Autodesk Inventor part; units mm, degrees
ref_plane "YZ Plane" through (0, 0, 0) normal (1, 0, 0) x (0, 1, 0)
ref_plane "XZ Plane" through (0, 0, 0) normal (0, 1, 0) x (-1, 0, 0)
ref_plane "XY Plane" through (0, 0, 0) normal (0, 0, 1) x (1, 0, 0)
sketch "スケッチ1" plane through (0, 0, 0) normal (0, 1, 0) x (-1, 0, 0)
  line L0 (5.0263, 6.4044) -> (-44.9737, 6.4044)
  line L1 (-44.9737, 6.4044) -> (-44.9737, -43.5956)
  line L2 (-44.9737, -43.5956) -> (5.0263, -43.5956)
  line L3 (5.0263, -43.5956) -> (5.0263, 6.4044)
  point P0 (0, 0)
  dimension "d0" = 50
  dimension "d1" = 50
extrude "押し出し1" add sketch "スケッチ1" along normal blind 2
sketch "スケッチ2" plane through (0, 2, 0) normal (0, 1, 0) x (1, 0, 0)
  circle A0 centre (19.9737, 1.0956) radius 1.5
  line L0 (-5.0263, -6.4044) -> (44.9737, -6.4044)
  line L1 (-5.0263, 43.5956) -> (-5.0263, -6.4044)
  circle A1 centre (9.9737, 1.0956) radius 1.5
  circle A2 centre (29.9737, 1.0956) radius 1.5
  circle A3 centre (9.9737, 18.5956) radius 1.5
  circle A4 centre (19.9737, 18.5956) radius 1.5
  circle A5 centre (29.9737, 18.5956) radius 1.5
  point P0 (0, 0)
  dimension "d4" = 3
  dimension "d5" = 7.5
  dimension "d6" = 25
  dimension "d7" = 3
  dimension "d8" = 3
  dimension "d9" = 10
  dimension "d10" = 10
  dimension "d11" = 3
  dimension "d12" = 17.5
  dimension "d13" = 3
  dimension "d14" = 3
  dimension "d15" = 10
  dimension "d16" = 10
  dimension "d17" = 17.5
hole "穴1" at (9.9737, 2, -1.0956) at (19.9737, 2, -1.0956) at (29.9737, 2, -1.0956) at (9.9737, 2, -18.5956) at (19.9737, 2, -18.5956) at (29.9737, 2, -18.5956) direction (0, -1, 0) diameter 3 depth 2
sketch "スケッチ3" plane through (0, 2, 0) normal (0, 1, 0) x (1, 0, 0)
  line L0 (-4.9253, -3.4044) -> (44.9737, -3.4044)
  line L1 (44.9737, -6.4044) -> (44.9737, 43.5956)
  line L2 (-5.0263, -6.4044) -> (44.9737, -6.4044)
  point P0 (0, 0)
  dimension "d25" = 3
sketch "スケッチ4" plane through (0, 2, 0) normal (0, 1, 0) x (1, 0, 0)
  line L0 (-5.0263, 43.5956) -> (-5.0263, -6.4044)
  line L1 (-5.0263, -6.4044) -> (44.9737, -6.4044)
  line L2 (-5.0263, -6.4044) -> (44.9737, -6.4044)
  line L3 (44.9737, -6.4044) -> (44.9737, -3.4044)
  line L4 (44.9737, -6.4044) -> (44.9737, 43.5956)
  line L5 (44.9737, -3.4044) -> (-5.0263, -3.4044)
  line L6 (-5.0263, -3.4044) -> (-5.0263, -6.4044)
  point P0 (0, 0)
  dimension "d26" = 3
extrude "押し出し2" cut sketch "スケッチ4" against normal blind 10
sketch "スケッチ5" plane through (0, 2, 0) normal (0, 1, 0) x (1, 0, 0)
  circle A0 centre (9.9737, 1.0956) radius 1.6
  line L0 (-5.0263, -3.4044) -> (44.9737, -3.4044)
  circle A1 centre (9.9737, 18.5956) radius 1.5
  circle A2 centre (9.9737, 18.5956) radius 1.6
  circle A3 centre (19.9737, 18.5956) radius 1.6
  circle A4 centre (19.9737, 1.0956) radius 1.6
  circle A5 centre (29.9737, 18.5956) radius 1.6
  circle A6 centre (29.9737, 1.0956) radius 1.6
  line L1 (-5.0263, 43.5956) -> (-5.0263, -3.4044)
  point P0 (0, 0)
  dimension "d29" = 3.2
  dimension "d30" = 4.5
  dimension "d32" = 3.2
  dimension "d33" = 3.2
  dimension "d34" = 3.2
  dimension "d35" = 3.2
  dimension "d36" = 3.2
  dimension "d37" = 4.5
  dimension "d38" = 17.5
  dimension "d39" = 17.5
  dimension "d40" = 17.5
  dimension "d41" = 4.5
  dimension "d42" = 10
  dimension "d43" = 10
  dimension "d44" = 10
  dimension "d45" = 15
  dimension "d46" = 15
  dimension "d47" = 10
hole "穴2" at (9.9737, 2, -1.0956) at (19.9737, 2, -1.0956) at (29.9737, 2, -1.0956) at (29.9737, 2, -18.5956) at (19.9737, 2, -18.5956) at (9.9737, 2, -18.5956) direction (0, -1, 0) diameter 3.2 depth 3
equation "\"BendRadius\" = Thickness"
equation "\"BendReliefWidth\" = Thickness"
equation "\"BendReliefDepth\" = 0.5 * Thickness"
equation "\"CornerReliefSize\" = 4 * Thickness"
equation "\"MinimumRemnant\" = 2 * Thickness"
equation "\"TransitionRadius\" = BendRadius"
equation "\"JacobiRadiusSize\" = BendRadius"
equation "\"GapSize\" = Thickness"
properties part number "nhk20" material "アルミニウム 6061"
Could you check a few things on this model? Use its own coordinates, in mm. Coordinates: 2 decimals unless noted, no trailing zeros. Order: outer loops, then holes, each group sorted by start corner. A loop starts at its lowest first (then second) coordinate and runs counter-clockwise, first axis right, second up.
Q1. Suppose I cut it at A-A on z = -1.5. Please give me the cut outline in (x, y), and give its area (3 significant figures).
Q2. Will this pin go through, and if not, where does the flat tip stop? pin 1 (4 mm diameter, centred on x = 39, z = -21.5, fed in from -Y).
Q3. Thinking about a two-plate mould opening in X: for faces 1 (the flat face through (-5.026, 1, -20)), 2 (the cylindrical face through (18.62, 0.99, -17.74)), 3 (the flat face through (20, 1, -43.596)), 4 (the cylindrical face through (11.393, 0.986, -17.857)), which applies, released by +X, released by -X, zero draft, split by the parting line, or undercut?
Q4. Suppose I cut it at B-B on y = 1.25. Please give me the cut outline in (x, z), and give its area (3 significant figures).
Q5. Please list where this line runs through material, in increasing order: L1, parallel to Z at x = 31, y = 1.55.
Q6. Suppose I cut it at D-D on z = -18.5. Please give me the cut outline in (x, y), and give its area (3 significant figures).
Q7. Suppose I cut it at C-C on x = 31. Please give me the cut outline in (y, z), and give its area (3 significant figures).
Answer:
1. outline: (-5.03, 0) - (8.43, 0) - (8.43, 2) - (-5.03, 2) - close; (11.52, 0) - (18.43, 0) - (18.43, 2) - (11.52, 2) - close; (21.52, 0) - (28.43, 0) - (28.43, 2) - (21.52, 2) - close; (31.52, 0) - (44.97, 0) - (44.97, 2) - (31.52, 2) - close
1. area: 81.4 mm2
2. pin 1: stops at y = 0
3. face 1: released by -X
3. face 2: undercut
3. face 3: zero draft
3. face 4: undercut
4. outline: (-5.03, -43.6) - (44.97, -43.6) - (44.97, 3.4) - (-5.03, 3.4) - close; hole circle Ø3.2 at (9.97, -18.6); hole circle Ø3.2 at (9.97, -1.1); hole circle Ø3.2 at (19.97, -18.6); hole circle Ø3.2 at (19.97, -1.1); hole circle Ø3.2 at (29.97, -18.6); hole circle Ø3.2 at (29.97, -1.1)
4. area: 2,300 mm2
5. L1: z = -43.6 to -19.82, -17.37 to -2.32, 0.13 to 3.4
6. outline: (-5.03, 0) - (8.38, 0) - (8.38, 2) - (-5.03, 2) - close; (11.57, 0) - (18.38, 0) - (18.38, 2) - (11.57, 2) - close; (21.57, 0) - (28.38, 0) - (28.38, 2) - (21.57, 2) - close; (31.57, 0) - (44.97, 0) - (44.97, 2) - (31.57, 2) - close
6. area: 80.8 mm2
7. outline: (0, -43.6) - (2, -43.6) - (2, -19.82) - (0, -19.82) - close; (0, -17.37) - (2, -17.37) - (2, -2.32) - (0, -2.32) - close; (0, 0.13) - (2, 0.13) - (2, 3.4) - (0, 3.4) - close
7. area: 84.2 mm2
